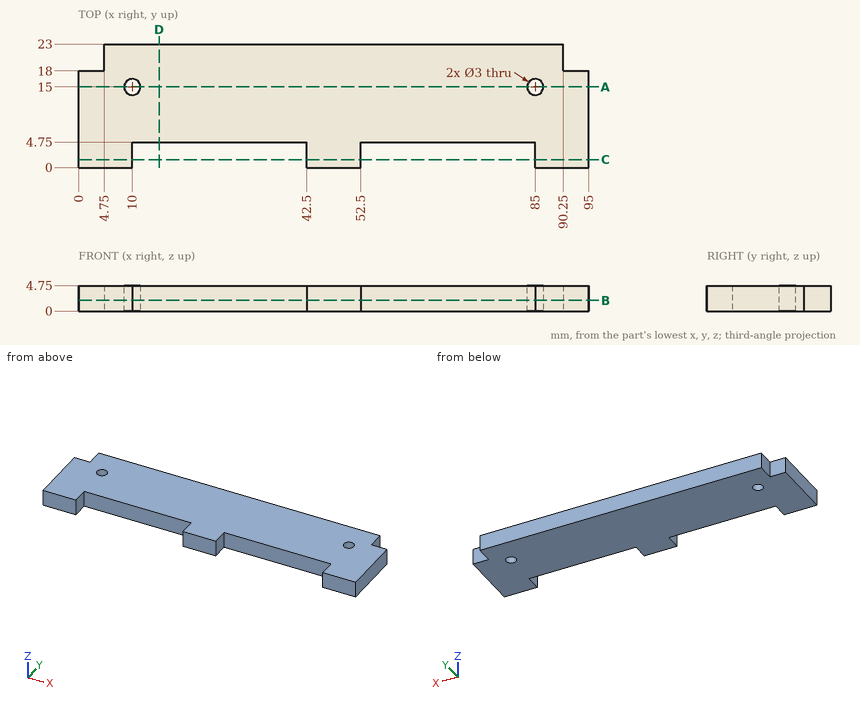
The figure shows three views and two pictorial views of one solid part (mm, origin at its lowest corner). Answer the questions. Give positions to 0.01 mm unless a question says otherwise; leave off trailing zeros. Order: outer loops, then holes, each group sorted by start corner. A loop starts at its lowest first (then second) coordinate and runs counter-clockwise, first axis right, second up. Notation, with made-up numbers: (-4, 5.25) - (45, 5.25) arc R16 cw to (45, 23.25) - close; hole circle Ø7 at (12.25, 62.25). An arc over 180 degrees is marked (long way). Answer as CSV lines item,"result".
Q1. A cutting plane is placed at A-A, the plane y = 15. Determine the outline of the cut face in (x, z), and give its area (3 significant figures).
Answer key:
outline,"(0, 0) - (8.5, 0) - (8.5, 4.75) - (0, 4.75) - close; (11.5, 0) - (83.5, 0) - (83.5, 4.75) - (11.5, 4.75) - close; (86.5, 0) - (95, 0) - (95, 4.75) - (86.5, 4.75) - close"
area,"423 mm^2"
Q2. A cutting plane is placed at D-D, the plane x = 15. Determine the outline of the cut face in (y, z).
Answer key:
outline,"(4.75, 0) - (23, 0) - (23, 4.75) - (4.75, 4.75) - close"
Q3. Straight lines are drawn through the part: L1, parallel to X at y = 1.5, z = 3.1; L2, parallel to X at y = 15.75, z = 1.3; L3, parallel to Y at x = 68, z = 3.6. For each, find the intervals that lie inside material, in ascending order.
Answer key:
L1,"x = 0 to 10, 42.5 to 52.5, 85 to 95"
L2,"x = 0 to 8.7, 11.3 to 83.7, 86.3 to 95"
L3,"y = 4.75 to 23"
Q4. Each of these flat-tipped pins is pushed along its axis until it touches: pin 1 Ø5 at (x, y) = (73, 5.5) entering from -Z; pin 2 Ø2.5 at (y, z) = (20, 1.5) entering from +X; pin 3 Ø2.5 at (x, z) = (68.5, 3.5) entering from -Y; pin 4 Ø1.4 at (x, z) = (2, 1.5) entering from +Y. Where does it stop, or does it pass through?
Answer key:
pin 1,"stops at z = 0"
pin 2,"stops at x = 90.25"
pin 3,"stops at y = 4.75"
pin 4,"stops at y = 18"
Q5. A cutting plane is placed at C-C, the plane y = 1.5. Determine the outline of the cut face in (x, z), and give its area (4 significant figures).
Answer key:
outline,"(0, 0) - (10, 0) - (10, 4.75) - (0, 4.75) - close; (42.5, 0) - (52.5, 0) - (52.5, 4.75) - (42.5, 4.75) - close; (85, 0) - (95, 0) - (95, 4.75) - (85, 4.75) - close"
area,"142.5 mm^2"
Q6. A cutting plane is placed at B-B, the plane z = 2. Determine the outline of the cut face in (x, y), and give its area (3 significant figures).
Answer key:
outline,"(0, 0) - (10, 0) - (10, 4.75) - (42.5, 4.75) - (42.5, 0) - (52.5, 0) - (52.5, 4.75) - (85, 4.75) - (85, 0) - (95, 0) - (95, 18) - (90.25, 18) - (90.25, 23) - (4.75, 23) - (4.75, 18) - (0, 18) - close; hole circle Ø3 at (10, 15); hole circle Ø3 at (85, 15)"
area,"1,810 mm^2"
